Design review of the part built by this model. Coordinates are the model's own, in mm. Face numbers are marked on the shaded views. A direction names the side the tool comes from. Coordinates: 2 decimals unless noted, no trailing zeros. Loops run counter-clockwise (first coordinate to the right, second up) from the corner with the lowest first, then second, coordinate; pieces in that order, holes last. Notation, with made-up numbers: (-19.5, -5.5) -> (1.5, -5.5) arc R11 cw to (1.5, 11.5) -> close; hole circle Ø9 at (-35, 47.25). An arc over 180 degrees is marked (long way). Use one line per item in the form item = value. Start each with the question number.
1. Machinability: for the marked faces 1 and 2, which of the approach directions +Z, -Z, +X, -X, +Y, -Y give a long, thin tool a straight path to every point of the face, cutting with its end or side? Answer none if there is none.
2. Wall thickness on line 1 (Z direction, x = -5.5, y = 1.75); line 2 (X direction, y = 0.25, z = -6.5); line 3 (X direction, y = 6.25, z = -6): over which ranges is each line inside the solid? List them lowest first. Write a range as from..to.
3. Consider section C-C (z = -6.5). State the section outline as (x, y) points, then the cut area to 3 significant figures.
4. For pin 1 (1.5 mm diameter, centred on y = -1, z = -5.5, fed in from +X); pin 2 (3 mm diameter, centred on y = -3.5, z = 5.5, fed in from +X); pin 3 (1.5 mm diameter, centred on x = -2, z = 0.5, fed in from +Y), all flat-tipped, find the tip position at first contact; note any pin that passes through.
5. Consider section D-D (z = 1). State the section outline as (x, y) points, then the cut area to 3 significant figures.
6. Consider section A-A (y = 0). State the section outline as (x, z) points.
from build123d import *

# Parameters (mm, degrees)
SKETCH1_R           = 4.8
BOSS_EXTRUDE1_DEPTH = 8.9
FILLET1_R           = 0.8
SKETCH2_R           = 7
BOSS_EXTRUDE2_DEPTH = 4


with BuildPart() as part:
    # Sketch1 → Boss-Extrude1 (new body, symmetric)
    with BuildSketch(Plane.XY):
        Circle(SKETCH1_R)
    extrude(amount=BOSS_EXTRUDE1_DEPTH, both=True)

    # Fillet1
    fillet1_edges = [part.edges().sort_by_distance(p)[0] for p in [
        (-4.8, 0, 8.9),
    ]]
    fillet(fillet1_edges, radius=FILLET1_R)

    # Sketch2 → Boss-Extrude2 (add)
    with BuildSketch(Plane(origin=(0, 0, -8.9), x_dir=(-1, 0, 0), z_dir=(0, 0, -1))):
        Circle(SKETCH2_R)
    extrude(amount=-BOSS_EXTRUDE2_DEPTH)


solid = part.part
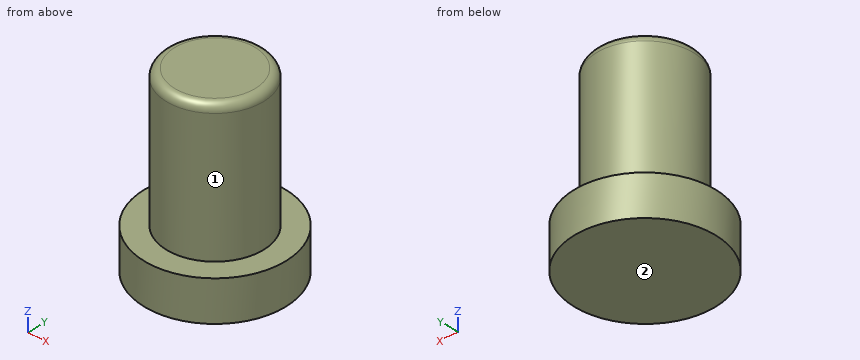
Geometry check:
q1.face_1 = +Z
q1.face_2 = -Z, +X, -X, +Y, -Y
q2.line_1 = -8.9..-4.9
q2.line_2 = -7..7
q2.line_3 = -3.15..3.15
q3.outline = circle Ø14 at (0, 0)
q3.area = 154 mm²
q4.pin_1 = 7
q4.pin_2 = 4.36
q4.pin_3 = 4.63
q5.outline = circle Ø9.6 at (0, 0)
q5.area = 72.4 mm²
q6.outline = (-7, -8.9) -> (7, -8.9) -> (7, -4.9) -> (4.8, -4.9) -> (4.8, 8.1) arc R0.8 ccw to (4, 8.9) -> (-4, 8.9) arc R0.8 ccw to (-4.8, 8.1) -> (-4.8, -4.9) -> (-7, -4.9) -> close
